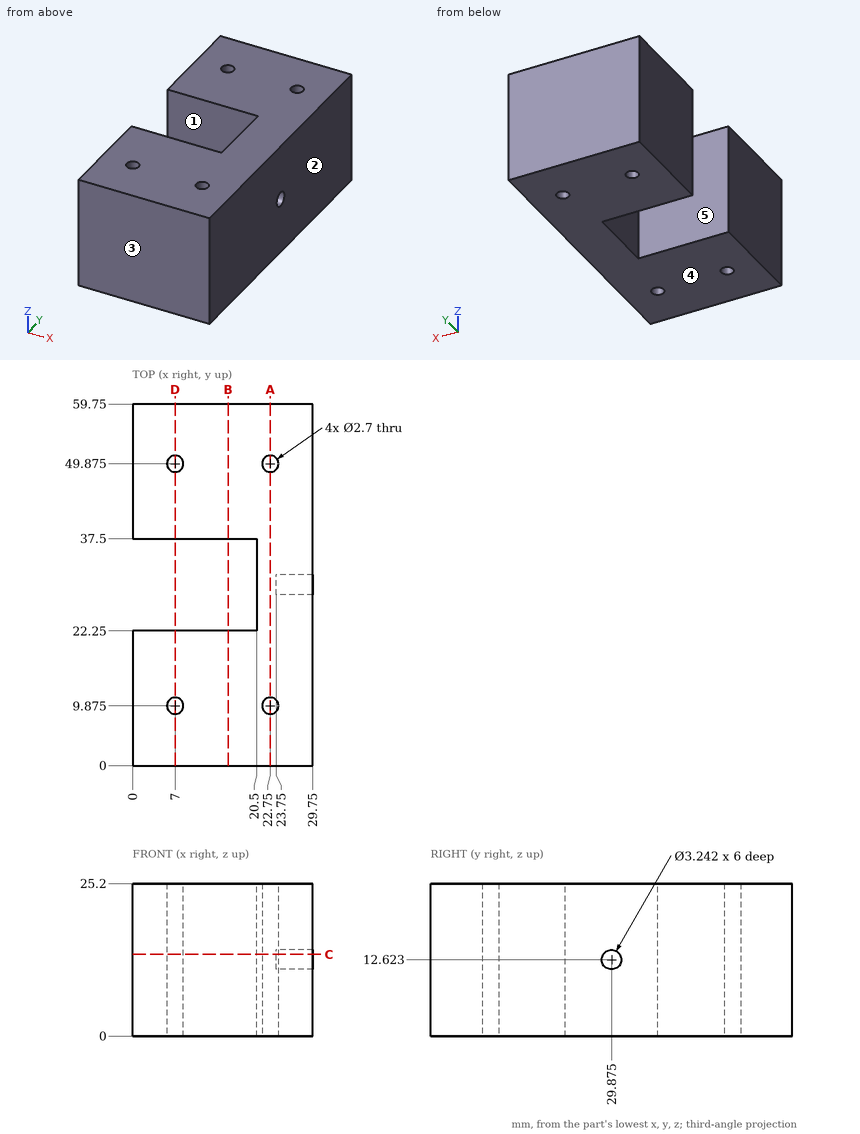
Print and shaded views of the part. All mm, measured from the part's lowest x, y and z. A direction names the side the tool comes from. Give positions to 0.01 mm unless a question says otherwise; leave off trailing zeros. Order: outer loops, then holes, each group sorted by start corner. A loop starts at its lowest first (then second) coordinate and runs counter-clockwise, first axis right, second up. Notation, with made-up numbers: (-14.5, 8) - (19.5, 8) arc R25 ccw to (19.5, 37) - close; hole circle Ø10 at (3, 26). An arc over 180 degrees is marked (long way). One line per item, written item: value.
Item 1: Tool access for the marked faces 1 and 2: list every direction of +Z, -Z, +X, -X, +Y, -Y with a clear straight run to the whole face (end or side of a thin tool).
Response values:
face 1: +Z, -Z, -X
face 2: +Z, -Z, +X, +Y, -Y
Item 2: Wall check: line 1 (Y direction, x = 22.75, z = 1.75) (3 decimals); line 2 (Y direction, x = 7, z = 13.5) (3 decimals); line 3 (X direction, y = 49.5, z = 6.5). Give the ranges that are in metal, low to high.
Response values:
line 1: 0 to 8.525, 11.225 to 48.525, 51.225 to 59.75
line 2: 0 to 8.525, 11.225 to 22.25, 37.5 to 48.525, 51.225 to 59.75
line 3: 0 to 5.7, 8.3 to 21.45, 24.05 to 29.75
Item 3: Two-plate mould, pull along Y, no slides. Class the marked faces 3, 4 and 5: released by +Y, released by -Y, zero draft, split by the parting line, or undercut.
Response values:
face 3: released by -Y
face 4: zero draft
face 5: undercut
Item 4: Pin check, flat tips, straight feed: pin 1 Ø2.5 at (y, z) = (29.88, 12.62) entering from +X; pin 2 Ø1.6 at (x, y) = (22.75, 49.875) entering from +Z; pin 3 Ø4.5 at (y, z) = (32, 18.5) entering from -X. Stop position of each tip, or through.
Response values:
pin 1: x = 23.75
pin 2: through
pin 3: x = 20.5
Item 5: Slice it at D-D (x = 7). List the corners of the cut face in (y, z) (3 decimals), then the cut area to 3 significant figures.
Response values:
outline: (0, 0) - (8.525, 0) - (8.525, 25.2) - (0, 25.2) - close; (11.225, 0) - (22.25, 0) - (22.25, 25.2) - (11.225, 25.2) - close; (37.5, 0) - (48.525, 0) - (48.525, 25.2) - (37.5, 25.2) - close; (51.225, 0) - (59.75, 0) - (59.75, 25.2) - (51.225, 25.2) - close
area: 985 mm2
Item 6: Slice it at B-B (x = 15.75). List the corners of the cut face in (y, z), then the cut area to 3 significant figures.
Response values:
outline: (0, 0) - (22.25, 0) - (22.25, 25.2) - (0, 25.2) - close; (37.5, 0) - (59.75, 0) - (59.75, 25.2) - (37.5, 25.2) - close
area: 1,120 mm2
Item 7: Slice it at A-A (x = 22.75). List the corners of the cut face in (y, z) (3 decimals).
Response values:
outline: (0, 0) - (8.525, 0) - (8.525, 25.2) - (0, 25.2) - close; (11.225, 0) - (48.525, 0) - (48.525, 25.2) - (11.225, 25.2) - close; (51.225, 0) - (59.75, 0) - (59.75, 25.2) - (51.225, 25.2) - close
Item 8: Slice it at C-C (z = 13.5). Give the number of separate pieces and of enclosed holes in the cut face, then the cut area to 3 significant figures.
Response values:
separate pieces: 1
enclosed holes: 4
area: 1,430 mm2
